Part print with two shaded views. Sizes in mm from the minimum x, y, z corner. A direction names the side the tool comes from. Round coordinates to 2 decimals unless told otherwise and drop trailing zeros. One line per question, with ' | ' between items.
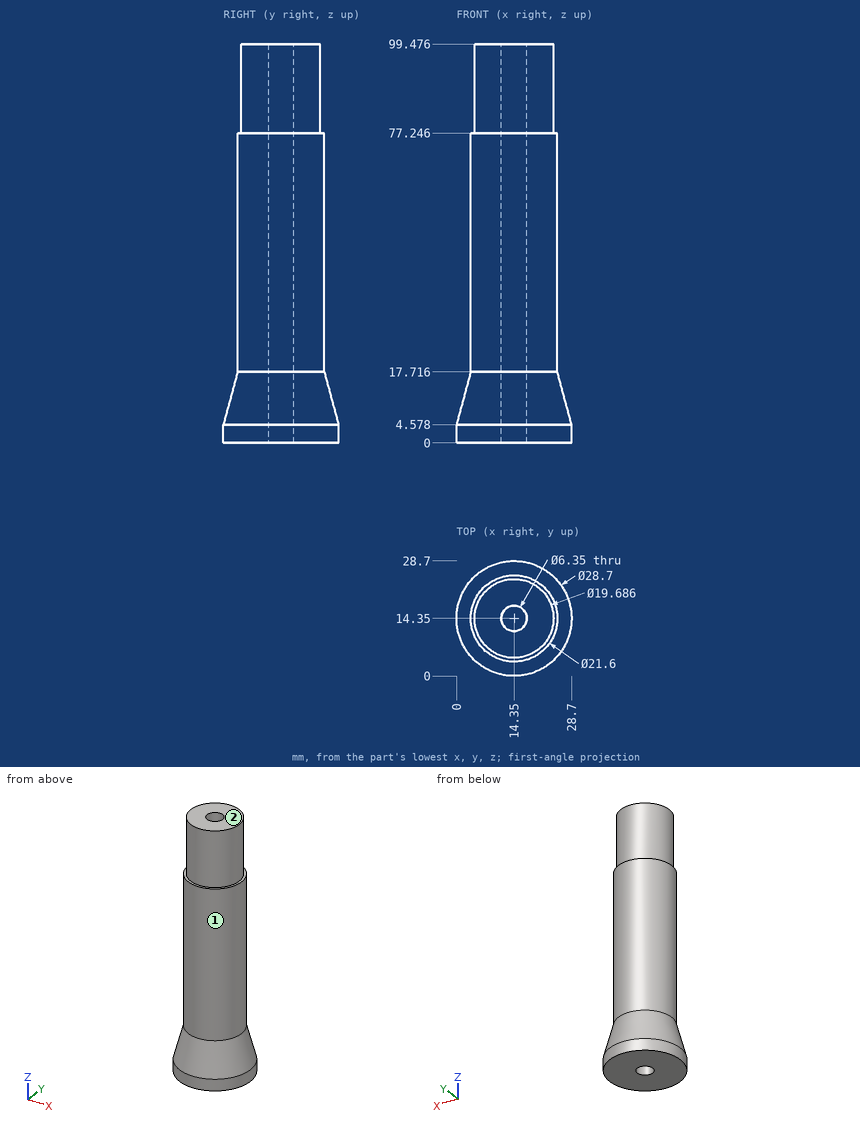
1) Which spindle directions (+Z, -Z, +X, -X, +Y, -Y) get a long thin tool onto all of the face, cutting with end or side? Do the marked faces 1 and 2. Say none if no direction does.
The answers:
face 1: +Z | face 2: +Z, +X, -X, +Y, -Y
2) Drop flat-ended pins along their axis: pin 1 (4 mm diameter, centred on x = 12.5, z = 79.5, fed in from +Y); pin 2 (6 mm diameter, centred on y = 6, z = 86, fed in from -X); pin 3 (8 mm diameter, centred on y = 14.5, z = 81, fed in from +X). Give the stop position or say it passes through.
The answers:
pin 1: stops at y = 24.19 | pin 2: stops at x = 6.09 | pin 3: stops at x = 25.15
3) Probe line 1 (Y direction, x = 14.25, z = 63.5); line 2 (Y direction, x = 6.75, z = 52) (1 decimal); line 3 (Y direction, x = 8.75, z = 62.5) (1 decimal). List the from-to ranges inside material, lowest first. Write a range as [from, to].
The answers:
line 1: y = [3.55, 11.18], [17.52, 25.15] | line 2: y = [6.7, 22] | line 3: y = [5.1, 23.6]
